Design review of the part shown in the three views and the two pictorial views. Dimensions are in mm from the part's minimum x, y and z. Coordinates: 2 decimals unless noted, no trailing zeros. Write each loop counter-clockwise with the first axis right and the second up, starting at its lowest first coordinate (ties: lowest second). Pieces come first, ordered by that corner, then holes. Notation, with made-up numbers: (87.5, 45) -> (135.5, 45) arc R32 ccw to (135.5, 71) -> close; hole circle Ø8 at (9.25, 2.25). An arc over 180 degrees is marked (long way). Write item = value, one per line. Start each with the question number.
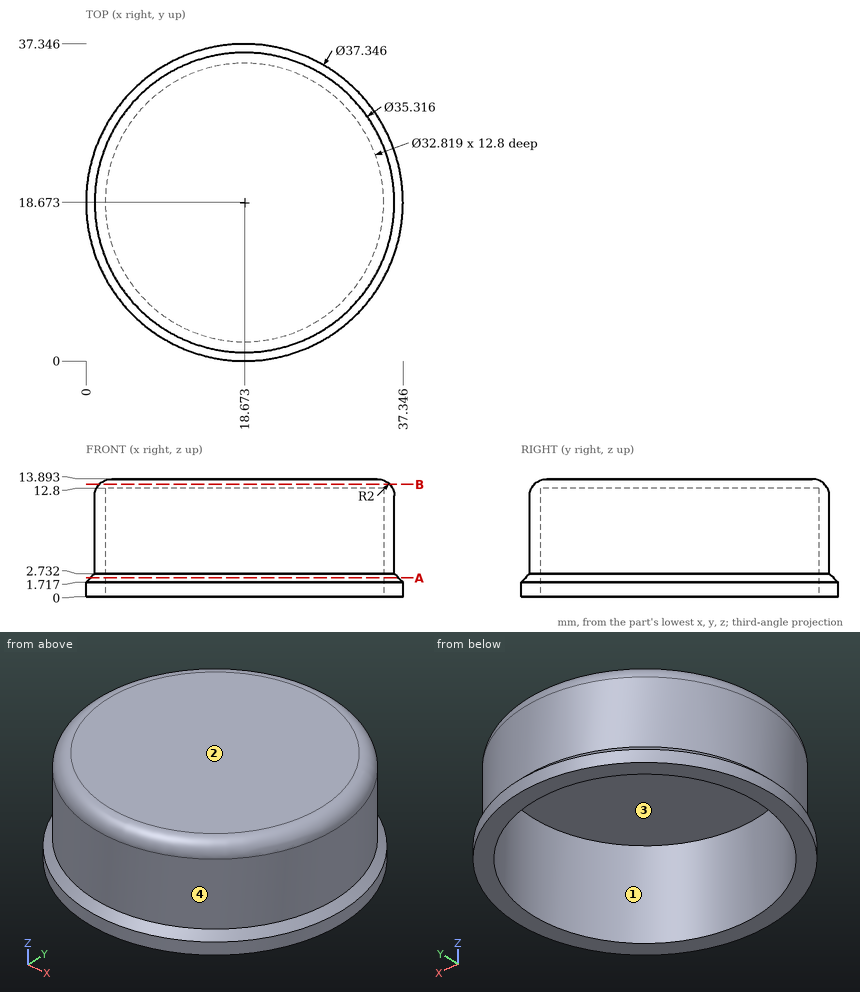
(1) For line 1 (X direction, y = 19, z = 10.5); line 2 (X direction, y = 27, z = 11) (1 decimal); line 3 (Y direction, x = 28.5, z = 3) (1 decimal), list the stretches that pass through material, from the lowest coordinate up.
(2) For pin 1 Ø1.5 at (x, z) = (29, 6.5) entering from -Y; pin 2 Ø2 at (x, z) = (5.5, 9.5) entering from -Y; pin 3 Ø6 at (x, z) = (8.5, 2.5) entering from +Y, all flat-tipped, find the tip position at first contact; note any pin that passes through.
(3) Mouldability with a two-part tool opening along X and no side actions: class the marked faces 1, 2, 3 and 4 as pulls with the +X half, pulls with the -X half, needs draft (parallel to the pull), parting line crosses it, or undercut.
(4) Take a section at B-B, the plane z = 13.25. State the section outline as (x, y) points.
(5) Take a section at A-A, the plane z = 2.25. State the section outline as (x, y) points.
Report:
q1.line_1 = 1.02 to 2.27, 35.08 to 36.33
q1.line_2 = 3.1 to 4.5, 32.8 to 34.2
q1.line_3 = 4 to 5.5, 31.8 to 33.3
q2.pin_1 = 3.84
q2.pin_2 = 5.88
q2.pin_3 = 35.87
q3.face_1 = undercut
q3.face_2 = needs draft
q3.face_3 = undercut
q3.face_4 = parting line crosses it
q4.outline = circle Ø34.25 at (18.67, 18.67)
q5.outline = circle Ø36.28 at (18.67, 18.67); hole circle Ø32.82 at (18.67, 18.67)
